Input: part model. Units: mm. Frame: model coordinates. A direction names the side the tool comes from. Round coordinates to 2 decimals unless told otherwise and drop trailing zeros. Write each loop counter-clockwise with the first axis right and the second up, starting at its lowest first coordinate (ties: lowest second). Pieces come first, ordered by that corner, then holes. Notation, with made-up numbers: (-5.5, 16) - (37.5, 16) arc R15 cw to (37.5, 40) - close; hole circle Ø3 at (62.25, 24.5). An arc over 180 degrees is marked (long way). One line per item, written item: value. Start each with the question number.
```python
from build123d import *

# Parameters (mm, degrees)
BOSS_EXTRUDE1_DEPTH = 3.175
SKETCH2_R           = 4.7625
BOSS_EXTRUDE2_DEPTH = 2.23012
BOSS_EXTRUDE3_DEPTH = 1.5


with BuildPart() as part:
    # Sketch1 → Boss-Extrude1 (new body)
    with BuildSketch(Plane(origin=(0, 0, 0), x_dir=(1, 0, 0), z_dir=(0, 1, 0))):
        Polygon((1.374815329, 2.38125), (-1.374815329, 2.38125), (-2.749630657, 0), (-1.374815329, -2.38125), (1.374815329, -2.38125), (2.749630657, 0), align=None)
    extrude(amount=BOSS_EXTRUDE1_DEPTH)

    # Sketch2 → Boss-Extrude2 (add)
    with BuildSketch(Plane(origin=(0, 3.175, 0), x_dir=(1, 0, 0), z_dir=(0, 1, 0))):
        Circle(SKETCH2_R)
    extrude(amount=BOSS_EXTRUDE2_DEPTH)

    # Sketch3 → Boss-Extrude3 (add)
    with BuildSketch(Plane(origin=(0, 5.40512, 0), x_dir=(1, 0, 0), z_dir=(0, 1, 0))):
        with BuildLine():
            Line((-2.347338919, 0.5), (2.347338919, 0.5))
            ThreePointArc((2.347338919, 0.5), (2.4, 0), (2.347338919, -0.5))
            Line((2.347338919, -0.5), (-2.347338919, -0.5))
            ThreePointArc((-2.347338919, -0.5), (-2.4, 0), (-2.347338919, 0.5))
        make_face()
    extrude(amount=BOSS_EXTRUDE3_DEPTH)


solid = part.part
```
Q1. Cut plane A-A, the plane x = 0. Output: boundary loops of the cut face in (y, z) (1 decimal).
Q2. Cut plane B-B, the plane y = 3. Output: boundary loops of the cut face in (x, z), and give its area (3 significant figures).
Q3. Cut plane D-D, the plane x = -2. Output: boundary loops of the cut face in (y, z) (3 decimals).
Q4. Access query for faces 1 (the flat face through (0, 2, -2.381)), 2 (the flat face through (-2.05, 1.57, -1.21)), 3 (the cylindrical face through (2.4, 6.1, 0)), 4 (the flat face through (0, 6, -0.5)), 5 (the flat face through (2, 3.175, 2)). Directions: +Z, -Z, +X, -X, +Y, -Y. A direction counts if a zero-diameter tool reaches every point of the face in a straight line with its end or side. Return the directions, or none.
Q5. Material intervals for probe 1 along Y at (x, z) = (3, -0.5) (3 decimals); probe 2 along Y at (x, z) = (0.75, 2); probe 3 along Z at (x, y) = (-0.25, 6), sorted ascending. Write a range as from..to.
Q6. Cut plane C-C, the plane z = -1.75. Output: boundary loops of the cut face in (x, y) (3 decimals).
Q7. Contact query for flat-ended pins moving along their axis: pin 1 Ø1 at (x, y) = (1.5, 1) entering from +Z; pin 2 Ø1.5 at (x, y) = (-3, 4.5) entering from +Z; pin 3 Ø3 at (x, y) = (0, 1.5) entering from -Z. Output: stop coordinate, or through.
A:
1. outline: (0, -2.4) - (3.2, -2.4) - (3.2, -4.8) - (5.4, -4.8) - (5.4, -0.5) - (6.9, -0.5) - (6.9, 0.5) - (5.4, 0.5) - (5.4, 4.8) - (3.2, 4.8) - (3.2, 2.4) - (0, 2.4) - close
2. outline: (-2.75, 0) - (-1.37, -2.38) - (1.37, -2.38) - (2.75, 0) - (1.37, 2.38) - (-1.37, 2.38) - close
2. area: 19.6 mm²
3. outline: (0, -1.298) - (3.175, -1.298) - (3.175, -4.322) - (5.405, -4.322) - (5.405, -0.5) - (6.905, -0.5) - (6.905, 0.5) - (5.405, 0.5) - (5.405, 4.322) - (3.175, 4.322) - (3.175, 1.298) - (0, 1.298) - close
4. face 1: -Z, +X, -X, -Y
4. face 2: -Z, -X, -Y
4. face 3: +X, +Y
4. face 4: -Z, +X, -X, +Y
4. face 5: -Y
5. probe 1: y = 3.175..5.405
5. probe 2: y = 0..5.41
5. probe 3: z = -0.5..0.5
6. outline: (-4.429, 3.175) - (-1.739, 3.175) - (-1.739, 0) - (1.739, 0) - (1.739, 3.175) - (4.429, 3.175) - (4.429, 5.405) - (-4.429, 5.405) - close
7. pin 1: stops at z = 2.38
7. pin 2: stops at z = 4.2
7. pin 3: stops at z = -2.38
